```python
from build123d import *

# Parameters (mm, degrees)
SKETCH_R     = 25
PAD_DEPTH    = 58
SKETCH001_R  = 20
POCKET_DEPTH = 7
POCKET_TAPER = 20
FILLET_R     = 1


with BuildPart() as part:
    # Sketch → Pad (new body)
    with BuildSketch(Plane.XY):
        Circle(SKETCH_R)
    extrude(amount=PAD_DEPTH)

    # Sketch001 → Pocket (cut)
    with BuildSketch(Plane.XY.offset(58)):
        Circle(SKETCH001_R)
    extrude(amount=-POCKET_DEPTH, taper=POCKET_TAPER, mode=Mode.SUBTRACT)

    # Fillet
    fillet_edges = [part.edges().sort_by_distance(p)[0] for p in [
        (-25, 0, 58),
        (-25, 0, 0),
        (-20, 0, 58),
        (-17.452208, 0, 51),
    ]]
    fillet(fillet_edges, radius=FILLET_R)


solid = part.part
```
The listing builds one solid part. Answer for the finished solid, in the listing's coordinates (mm). Give positions to 0.01 mm unless a question says otherwise; leave off trailing zeros. Loops run counter-clockwise (first coordinate to the right, second up) from the corner with the lowest first, then second, coordinate; pieces in that order, holes last. Notation, with made-up numbers: (22.25, -26) - (42.25, -26) arc R8 ccw to (42.25, -16) - close; hole circle Ø10 at (57.5, 50). An arc over 180 degrees is marked (long way). Return JSON: item names as keys, results as strings. Group by question number.
1. Find section B-B (z = 27.5). Write down the section's boundary in (x, y).
2. Determine the mould class of faces 1 (the cylindrical face through (23.846, 7.509, 28.608)), 2 (the flat face through (-18, -11, 58)), 3 (the flat face through (0, 0, 51)) for opening direction X: pulls with the +X half, pulls with the -X half, needs draft (parallel to the pull), parting line crosses it, or undercut.
3. Given pin 1 Ø10 at (x, y) = (-16, 5.5) entering from -Z; pin 2 Ø12 at (x, z) = (20, 31.5) entering from +Y; pin 3 Ø5 at (y, z) = (-7, 22) entering from +X; pin 4 Ø10 at (x, y) = (-0.5, -0.5) entering from +Z, each flat-ended and moving along its own axis, determine where each tip first touches the part or whether it passes through.
4. Straight lines are drawn through the part: line 1 (X direction, y = -7, z = 48.5); line 2 (Z direction, x = -9, y = -5.5); line 3 (X direction, y = 12, z = 48.5). For each, find the intervals that lie inside material, in ascending order. Write a range as [from, to].
5. Find section A-A (x = 0). Write down the section's boundary in (y, z).
Verdict:
{
 "1": {"outline": "circle Ø50 at (0, 0)"},
 "2": {"face 1": "parting line crosses it", "face 2": "needs draft", "face 3": "undercut"},
 "3": {"pin 1": "stops at z = 0", "pin 2": "stops at y = 20.71", "pin 3": "stops at x = 24.59", "pin 4": "stops at z = 51"},
 "4": {"line 1": "x = [-24, 24]", "line 2": "z = [0, 51]", "line 3": "x = [-21.93, 21.93]"},
 "5": {"outline": "(-25, 1) arc R1 ccw to (-24, 0) - (24, 0) arc R1 ccw to (25, 1) - (25, 57) arc R1 ccw to (24, 58) - (20.7, 58) arc R1 ccw to (19.76, 57.34) - (17.69, 51.66) arc R1 cw to (16.75, 51) - (-16.75, 51) arc R1 cw to (-17.69, 51.66) - (-19.76, 57.34) arc R1 ccw to (-20.7, 58) - (-24, 58) arc R1 ccw to (-25, 57) - close"}
}
